```python
from build123d import *

# Parameters (mm, degrees)
SKETCH1_R           = 1.5
BOSS_EXTRUDE1_DEPTH = 3
SKETCH2_R           = 1.5
BOSS_EXTRUDE2_DEPTH = 1


with BuildPart() as part:
    # Sketch1 → Boss-Extrude1 (new body)
    with BuildSketch(Plane.XY):
        Polygon((-95.5, -40), (-95.5, 40), (-72.165476221, 63.334523779), (72.165476221, 63.334523779), (95.5, 40), (95.5, -40), (72.165476221, -63.334523779), (-72.165476221, -63.334523779), align=None)
        with Locations((-90.5, 29)):
            Circle(SKETCH1_R, mode=Mode.SUBTRACT)
        with Locations((-90.5, -29)):
            Circle(SKETCH1_R, mode=Mode.SUBTRACT)
        with Locations((90.5, -29)):
            Circle(SKETCH1_R, mode=Mode.SUBTRACT)
        with Locations((90.5, 29)):
            Circle(SKETCH1_R, mode=Mode.SUBTRACT)
    extrude(amount=BOSS_EXTRUDE1_DEPTH)

    # Sketch2 → Boss-Extrude2 (add)
    with BuildSketch(Plane(origin=(0, 0, 0), x_dir=(-1, 0, 0), z_dir=(0, 0, -1))):
        Polygon((-59.403736545, 32.5), (-46.062041549, 32.5), (-81.28908922, 54.21091078), (-86.376387001, 49.123612999), align=None)
        Polygon((-34.704188524, 25.5), (-46.062041549, 32.5), (-59.403736545, 32.5), (-48.045883519, 25.5), align=None)
        Polygon((-48.045883519, 25.5), (-59.403736545, 32.5), (-95.5, 32.5), (-95.5, 25.5), align=None)
        with Locations((-90.5, 29)):
            Circle(SKETCH2_R, mode=Mode.SUBTRACT)
        Polygon((34.704188524, 25.5), (46.062041549, 32.5), (-46.062041549, 32.5), (-34.704188524, 25.5), align=None)
        Polygon((59.403736545, 32.5), (46.062041549, 32.5), (34.704188524, 25.5), (48.045883519, 25.5), align=None)
        Polygon((86.376387001, 49.123612999), (81.28908922, 54.21091078), (46.062041549, 32.5), (59.403736545, 32.5), align=None)
        Polygon((95.5, 32.5), (59.403736545, 32.5), (48.045883519, 25.5), (95.5, 25.5), align=None)
        with Locations((90.5, 29)):
            Circle(SKETCH2_R, mode=Mode.SUBTRACT)
        Polygon((-6.670847498, 0), (0, 4.111334455), (-34.704188524, 25.5), (-48.045883519, 25.5), align=None)
        Polygon((48.045883519, 25.5), (34.704188524, 25.5), (0, 4.111334455), (6.670847498, 0), align=None)
        Polygon((6.670847498, 0), (0, 4.111334455), (-6.670847498, 0), (0, -4.111334455), align=None)
        Polygon((48.045883519, -25.5), (6.670847498, 0), (0, -4.111334455), (34.704188524, -25.5), align=None)
        Polygon((0, -4.111334455), (-6.670847498, 0), (-48.045883519, -25.5), (-34.704188524, -25.5), align=None)
        Polygon((-34.704188524, -25.5), (-48.045883519, -25.5), (-59.403736545, -32.5), (-46.062041549, -32.5), align=None)
        Polygon((-59.403736545, -32.5), (-48.045883519, -25.5), (-95.5, -25.5), (-95.5, -32.5), align=None)
        with Locations((-90.5, -29)):
            Circle(SKETCH2_R, mode=Mode.SUBTRACT)
        Polygon((34.704188524, -25.5), (-34.704188524, -25.5), (-46.062041549, -32.5), (46.062041549, -32.5), align=None)
        Polygon((59.403736545, -32.5), (48.045883519, -25.5), (34.704188524, -25.5), (46.062041549, -32.5), align=None)
        Polygon((95.5, -25.5), (48.045883519, -25.5), (59.403736545, -32.5), (95.5, -32.5), align=None)
        with Locations((90.5, -29)):
            Circle(SKETCH2_R, mode=Mode.SUBTRACT)
        Polygon((86.376387001, -49.123612999), (59.403736545, -32.5), (46.062041549, -32.5), (81.28908922, -54.21091078), align=None)
        Polygon((-46.062041549, -32.5), (-59.403736545, -32.5), (-86.376387001, -49.123612999), (-81.28908922, -54.21091078), align=None)
    extrude(amount=BOSS_EXTRUDE2_DEPTH)


solid = part.part
```
Here's how the part is built. I have some questions about the finished solid (model axes, mm). A direction names the side the tool comes from. Coordinates: 2 decimals unless noted, no trailing zeros. Write each loop counter-clockwise with the first axis right and the second up, starting at its lowest first coordinate (ties: lowest second). Pieces come first, ordered by that corner, then holes. Notation, with made-up numbers: M 34.5,16.25 L 88.5,16.25 A22 ccw 88.5,43.25 Z; hole C 40.5,1 d4. An arc over 180 degrees is marked long. Answer as CSV lines item,"result". Start each with the question number.
Q1. Suppose I cut it at D-D, the plane y = -16.5. List the corners of the cut face in (x, z) for me.
Q2. Suppose I cut it at A-A, the plane z = 1.9. List the corners of the cut face in (x, y) for me, then the cut area to 3 significant figures.
Q3. Suppose I cut it at C-C, the plane x = -20. List the corners of the cut face in (y, z) for me, then the cut area to 3 significant figures.
Q4. If we mould it in two halves opening along X, with no side actions, what happens to faces 6 (the flat face through (-81, 39, 0)), 7 (the flat face through (-95.5, -1, 1)), 8 (the flat face through (63.922, -43.507, -0.493))? For each: pulls with the +X half, pulls with the -X half, needs draft (parallel to the pull), parting line crosses it, or undercut.
Q5. I need wall thicknesses on probe 1 along Y at (x, z) = (-90.5, -0.5); probe 2 along X at (y, z) = (-29, 2); probe 3 along Y at (x, z) = (90.5, 1.4). Which ranges of each line are inside material? Lowest first, please. Write a range as [from, to].
Q6. For faces 1 (the flat face through (-81, -39, 0)), 2 (the flat face through (84, -51.5, 1.5)), 3 (the flat face through (62, 0, 0)), 4 (the flat face through (1, 48, 0)), 5 (the flat face through (-17.6, 14.96, -0.49)), which set-ups out of +Z, -Z, +X, -X, +Y, -Y let a thin tool reach every point of the face, with its end or its side?
Q7. Suppose I cut it at B-B, the plane y = 43. List the corners of the cut face in (x, z) for me, then the cut area to 3 significant figures.
Q8. Will these pins go through, and if not, where does the flat tip stop? pin 1 Ø0.8 at (x, z) = (-3, -0.5) entering from +Y; pin 2 Ø0.5 at (x, z) = (-72, -0.5) entering from +Y; pin 3 Ø15.5 at (x, y) = (-6.5, -55) entering from -Z.
Entries:
1,outline,"M -95.5,0 L -33.44,0 L -33.44,-1 L -20.1,-1 L -20.1,0 L 20.1,0 L 20.1,-1 L 33.44,-1 L 33.44,0 L 95.5,0 L 95.5,3 L -95.5,3 Z"
2,outline,"M -95.5,-40 L -72.17,-63.33 L 72.17,-63.33 L 95.5,-40 L 95.5,40 L 72.17,63.33 L -72.17,63.33 L -95.5,40 Z; hole C -90.5,-29 d3; hole C -90.5,29 d3; hole C 90.5,-29 d3; hole C 90.5,29 d3"
2,area,"23,100 mm²"
3,outline,"M -63.33,0 L -32.5,0 L -32.5,-1 L -25.5,-1 L -25.5,0 L -16.44,0 L -16.44,-1 L -8.21,-1 L -8.21,0 L 8.21,0 L 8.21,-1 L 16.44,-1 L 16.44,0 L 25.5,0 L 25.5,-1 L 32.5,-1 L 32.5,0 L 63.33,0 L 63.33,3 L -63.33,3 Z"
3,area,"410 mm²"
4,face 6,"needs draft"
4,face 7,"pulls with the -X half"
4,face 8,"undercut"
5,probe 1,"y = [-32.5, -30.5], [-27.5, -25.5], [25.5, 27.5], [30.5, 32.5]"
5,probe 2,"x = [-95.5, -92], [-89, 89], [92, 95.5]"
5,probe 3,"y = [-45, -30.5], [-27.5, 27.5], [30.5, 45]"
6,face 1,"-Z, -X"
6,face 2,"+Z, -Z, +X, -Y"
6,face 3,"-Z, +X"
6,face 4,"-Z, +Y"
6,face 5,"-Z"
7,outline,"M -92.5,0 L -76.44,0 L -76.44,-1 L -63.1,-1 L -63.1,0 L 63.1,0 L 63.1,-1 L 76.44,-1 L 76.44,0 L 92.5,0 L 92.5,3 L -92.5,3 Z"
7,area,"582 mm²"
8,pin 1,"stops at y = 32.5"
8,pin 2,"stops at y = 48.64"
8,pin 3,"stops at z = 0"
